from build123d import *

# Parameters (mm, degrees)
SZKIC1_R                               = 4.5
DODANIE_WYCI_GNI_CIE1_DEPTH            = 8
SZKIC23_R                              = 6.5
WYTNIJ_WYCI_GNI_CIE11_DEPTH            = 5.5
SZKIC4_W                               = 8
SZKIC4_H                               = 40
DODANIE_WYCI_GNI_CIE2_DEPTH            = 62.15
DODANIE_WYCI_GNI_CIE3_DEPTH            = 8
WYTNIJ_WYCI_GNI_CIE3_REACH             = 91.171
SZKIC6_R                               = 1.6
SZKIC7_R                               = 3.75
WYTNIJ_WYCI_GNI_CIE4_DEPTH             = 3.5
WYTNIJ_WYCI_GNI_CIE5_REACH             = 97.976
WYTNIJ_WYCI_GNI_CIE5_DIRECTION_2_REACH = 97.976
SZKIC10_R                              = 3
WYTNIJ_WYCI_GNI_CIE6_DEPTH             = 2
WYTNIJ_WYCI_GNI_CIE7_REACH             = 93.888
SZKIC14_W                              = 8
SZKIC14_H                              = 62.15
DODANIE_WYCI_GNI_CIE5_DEPTH            = 78.15
WYTNIJ_WYCI_GNI_CIE9_DEPTH             = 215.763643338
WYTNIJ_WYCI_GNI_CIE9_DEPTH_BACK        = 215.763643338
SZKIC20_W                              = 10
SZKIC20_H                              = 20
WYTNIJ_WYCI_GNI_CIE10_DEPTH            = 5
ZAOKR_GLENIE1_R                        = 10
WYTNIJ_WYCI_GNI_CIE12_REACH            = 213.222
WYTNIJ_WYCI_GNI_CIE12_END_RADIUS       = 5
SZKIC24_R                              = 1.75
WYTNIJ_WYCI_GNI_CIE13_REACH            = 222.301
SZKIC25_R                              = 1.6


with BuildPart() as part:
    # Szkic1 → Dodanie-wyciągnięcie1 (new body)
    with BuildSketch(Plane(origin=(0, 0, 0), x_dir=(1, 0, 0), z_dir=(0, 1, 0))):
        Polygon((-14, -10), (30, -20), (38, -20), (38, 20), (30, 20), (-14, 10), align=None)
        with Locations(Location((0, 0, 0), (0, 0, 270))):
            Circle(SZKIC1_R, mode=Mode.SUBTRACT)
    extrude(amount=DODANIE_WYCI_GNI_CIE1_DEPTH)

    # Szkic23 → Wytnij-wyciągnięcie11 (cut)
    with BuildSketch(Plane.XZ):
        with Locations(Location((0, 0, 0), (0, 0, 270))):
            Circle(SZKIC23_R)
    extrude(amount=-WYTNIJ_WYCI_GNI_CIE11_DEPTH, mode=Mode.SUBTRACT)

    # Szkic4 → Dodanie-wyciągnięcie2 (add)
    with BuildSketch(Plane(origin=(0, 8, 0), x_dir=(1, 0, 0), z_dir=(0, 1, 0))):
        with Locations((34, 0)):
            Rectangle(SZKIC4_W, SZKIC4_H)
    extrude(amount=DODANIE_WYCI_GNI_CIE2_DEPTH)

    # Szkic5 → Dodanie-wyciągnięcie3 (add)
    with BuildSketch(Plane(origin=(0, 70.15, 0), x_dir=(1, 0, 0), z_dir=(0, 1, 0))):
        Polygon((38, -20), (38, 20), (30, 20), (-14, 10), (-14, -10), (30, -20), align=None)
    extrude(amount=DODANIE_WYCI_GNI_CIE3_DEPTH)

    # Szkic6 → Wytnij-wyciągnięcie3 (cut, up to next)
    with BuildSketch(Plane(origin=(0, 78.15, 0), x_dir=(1, 0, 0), z_dir=(0, 1, 0)), mode=Mode.PRIVATE) as wytnij_wyci_gni_cie3_sk1:
        with Locations(Location((-7, 0, 0), (0, 0, 270))):
            Circle(SZKIC6_R)
    wytnij_wyci_gni_cie3_tool1 = extrude(wytnij_wyci_gni_cie3_sk1.sketch, amount=-WYTNIJ_WYCI_GNI_CIE3_REACH, mode=Mode.PRIVATE) & part.part
    # Szkic6 → Wytnij-wyciągnięcie3 (cut, up to next)
    with BuildSketch(Plane(origin=(0, 78.15, 0), x_dir=(1, 0, 0), z_dir=(0, 1, 0)), mode=Mode.PRIVATE) as wytnij_wyci_gni_cie3_sk2:
        with Locations(Location((7, 0, 0), (0, 0, 270))):
            Circle(SZKIC6_R)
    wytnij_wyci_gni_cie3_tool2 = extrude(wytnij_wyci_gni_cie3_sk2.sketch, amount=-WYTNIJ_WYCI_GNI_CIE3_REACH, mode=Mode.PRIVATE) & part.part
    add(wytnij_wyci_gni_cie3_tool1.solids().sort_by_distance((-7, 78.15, 0))[0], mode=Mode.SUBTRACT)
    add(wytnij_wyci_gni_cie3_tool2.solids().sort_by_distance((7, 78.15, 0))[0], mode=Mode.SUBTRACT)

    # Szkic7 → Wytnij-wyciągnięcie4 (cut)
    with BuildSketch(Plane(origin=(0, 78.15, 0), x_dir=(1, 0, 0), z_dir=(0, 1, 0))):
        with Locations(Location((7, 0, 0), (0, 0, 270))):
            Circle(SZKIC7_R)
        with Locations(Location((-7, 0, 0), (0, 0, 270))):
            Circle(SZKIC7_R)
    extrude(amount=-WYTNIJ_WYCI_GNI_CIE4_DEPTH, mode=Mode.SUBTRACT)

    # Wytnij-wyciągnięcie5: up to this plane
    wytnij_wyci_gni_cie5_end = Plane(origin=(30, 78.15, -20), z_dir=(0.22162110358896817, 0, 0.9751328557914598))
    # Szkic9 → Wytnij-wyciągnięcie5 (cut, up to the surface)
    with BuildSketch(Plane(origin=(-14, 0, 0), x_dir=(1, 0, 0), z_dir=(0, 0, 1)), mode=Mode.PRIVATE) as wytnij_wyci_gni_cie5_sk1:
        with BuildLine():
            Line((10.5, 70.15), (17.5, 70.15))
            Line((17.5, 70.15), (17.5, 71.15))
            ThreePointArc((17.5, 71.15), (14, 72.579285786), (10.5, 71.15))
            Line((10.5, 71.15), (10.5, 70.15))
        make_face()
    wytnij_wyci_gni_cie5_tool1 = split(extrude(wytnij_wyci_gni_cie5_sk1.sketch, amount=-WYTNIJ_WYCI_GNI_CIE5_REACH, mode=Mode.PRIVATE), bisect_by=wytnij_wyci_gni_cie5_end, keep=Keep.BOTH, mode=Mode.PRIVATE)
    add(wytnij_wyci_gni_cie5_tool1.solids().sort_by_distance((0, 71.185303, 0))[0], mode=Mode.SUBTRACT)

    # Wytnij-wyciągnięcie5 direction 2: up to this plane
    wytnij_wyci_gni_cie5_direction_2_end = Plane(origin=(-14, 78.15, 10), z_dir=(0.22162110358896792, 0, -0.9751328557914598))
    # Szkic9 → Wytnij-wyciągnięcie5 direction 2 (cut, up to the surface)
    with BuildSketch(Plane(origin=(-14, 0, 0), x_dir=(1, 0, 0), z_dir=(0, 0, 1)), mode=Mode.PRIVATE) as wytnij_wyci_gni_cie5_direction_2_sk1:
        with BuildLine():
            Line((10.5, 70.15), (17.5, 70.15))
            Line((17.5, 70.15), (17.5, 71.15))
            ThreePointArc((17.5, 71.15), (14, 72.579285786), (10.5, 71.15))
            Line((10.5, 71.15), (10.5, 70.15))
        make_face()
    wytnij_wyci_gni_cie5_direction_2_tool1 = split(extrude(wytnij_wyci_gni_cie5_direction_2_sk1.sketch, amount=WYTNIJ_WYCI_GNI_CIE5_DIRECTION_2_REACH, mode=Mode.PRIVATE), bisect_by=wytnij_wyci_gni_cie5_direction_2_end, keep=Keep.BOTH, mode=Mode.PRIVATE)
    add(wytnij_wyci_gni_cie5_direction_2_tool1.solids().sort_by_distance((0, 71.185303, 0))[0], mode=Mode.SUBTRACT)

    # Szkic10 → Wytnij-wyciągnięcie6 (cut)
    with BuildSketch(Plane(origin=(0, 78.15, 0), x_dir=(1, 0, 0), z_dir=(0, 1, 0))):
        with Locations(Location((0, 0, 0), (0, 0, 270))):
            Circle(SZKIC10_R)
    extrude(amount=-WYTNIJ_WYCI_GNI_CIE6_DEPTH, mode=Mode.SUBTRACT)

    # Szkic14 → Wytnij-wyciągnięcie7 (cut, up to next)
    with BuildSketch(Plane.ZY.offset(-30), mode=Mode.PRIVATE) as wytnij_wyci_gni_cie7_sk1:
        with Locations((-16, 39.075)):
            Rectangle(SZKIC14_W, SZKIC14_H)
    wytnij_wyci_gni_cie7_tool1 = extrude(wytnij_wyci_gni_cie7_sk1.sketch, amount=-WYTNIJ_WYCI_GNI_CIE7_REACH, mode=Mode.PRIVATE) & part.part
    # Szkic14 → Wytnij-wyciągnięcie7 (cut, up to next)
    with BuildSketch(Plane.ZY.offset(-30), mode=Mode.PRIVATE) as wytnij_wyci_gni_cie7_sk2:
        with Locations((16, 39.075)):
            Rectangle(SZKIC14_W, SZKIC14_H)
    wytnij_wyci_gni_cie7_tool2 = extrude(wytnij_wyci_gni_cie7_sk2.sketch, amount=-WYTNIJ_WYCI_GNI_CIE7_REACH, mode=Mode.PRIVATE) & part.part
    add(wytnij_wyci_gni_cie7_tool1.solids().sort_by_distance((30, 39.075, -16))[0], mode=Mode.SUBTRACT)
    add(wytnij_wyci_gni_cie7_tool2.solids().sort_by_distance((30, 39.075, 16))[0], mode=Mode.SUBTRACT)

    # Szkic17 → Dodanie-wyciągnięcie5 (add, through all)
    with BuildSketch(Plane.XZ):
        Polygon((38, 20), (196, 12.5), (196, -12.5), (38, -20), (38, -11.990992093), (186, -4.965675637), (186, 4.965675637), (38, 11.990992093), align=None)
    extrude(amount=-DODANIE_WYCI_GNI_CIE5_DEPTH)

    # Szkic18 → Wytnij-wyciągnięcie9 (cut, two sides: drawn at the far end of the back side and taken through both)
    with BuildSketch(Plane(origin=(0, 0, -20), x_dir=(-1, 0, 0), z_dir=(0, 0, -1)).offset(-WYTNIJ_WYCI_GNI_CIE9_DEPTH_BACK)):
        Polygon((-196, 0), (-196, 19.075), (-38, 0), align=None)
        Polygon((-196, 59.075), (-196, 78.15), (-38, 78.15), align=None)
        Polygon((-38, 8), (-186, 25.867721519), (-186, 52.282278481), (-38, 70.15), align=None)
    extrude(amount=WYTNIJ_WYCI_GNI_CIE9_DEPTH + WYTNIJ_WYCI_GNI_CIE9_DEPTH_BACK, mode=Mode.SUBTRACT)

    # Szkic20 → Wytnij-wyciągnięcie10 (cut)
    with BuildSketch(Plane(origin=(196, 0, 0), x_dir=(0, 0, -1), z_dir=(1, 0, 0))):
        with Locations((0, 39.075)):
            Rectangle(SZKIC20_W, SZKIC20_H)
    extrude(amount=-WYTNIJ_WYCI_GNI_CIE10_DEPTH, mode=Mode.SUBTRACT)

    # Zaokrąglenie1
    zaokr_glenie1_edges = [part.edges().sort_by_distance(p)[0] for p in [
        (-14, 4, 10),
        (-14, 4, -10),
        (-14, 74.15, -10),
        (-14, 74.15, 10),
    ]]
    fillet(zaokr_glenie1_edges, radius=ZAOKR_GLENIE1_R)

    # Wytnij-wyciągnięcie12: up to this cylinder (the profile starts outside it)
    wytnij_wyci_gni_cie12_end = Plane(origin=(0, 67.579285786, 0), z_dir=(0, 0, -1)) * Cylinder(WYTNIJ_WYCI_GNI_CIE12_END_RADIUS, 437.444, mode=Mode.PRIVATE)
    # Szkic24 → Wytnij-wyciągnięcie12 (cut, up to the surface)
    with BuildSketch(Plane(origin=(0, 76.15, 0), x_dir=(1, 0, 0), z_dir=(0, 1, 0)), mode=Mode.PRIVATE) as wytnij_wyci_gni_cie12_sk1:
        with Locations(Location((0, 0, 0), (0, 0, 270))):
            Circle(SZKIC24_R)
    wytnij_wyci_gni_cie12_tool1 = extrude(wytnij_wyci_gni_cie12_sk1.sketch, amount=-WYTNIJ_WYCI_GNI_CIE12_REACH, mode=Mode.PRIVATE) - wytnij_wyci_gni_cie12_end
    add(wytnij_wyci_gni_cie12_tool1.solids().sort_by_distance((0, 76.15, 0))[0], mode=Mode.SUBTRACT)

    # Szkic25 → Wytnij-wyciągnięcie13 (cut, up to next)
    with BuildSketch(Plane(origin=(191, 0, 0), x_dir=(0, 0, -1), z_dir=(1, 0, 0)), mode=Mode.PRIVATE) as wytnij_wyci_gni_cie13_sk1:
        with Locations((0, 39.075)):
            Circle(SZKIC25_R)
    wytnij_wyci_gni_cie13_tool1 = extrude(wytnij_wyci_gni_cie13_sk1.sketch, amount=-WYTNIJ_WYCI_GNI_CIE13_REACH, mode=Mode.PRIVATE) & part.part
    add(wytnij_wyci_gni_cie13_tool1.solids().sort_by_distance((191, 39.075, 0))[0], mode=Mode.SUBTRACT)


solid = part.part
Source: CAD feature listing. Evaluate the final solid. Frame: model axes, mm. A direction names the side the tool comes from. Give positions to 0.01 mm unless a question says otherwise; leave off trailing zeros. Write each loop counter-clockwise with the first axis right and the second up, starting at its lowest first coordinate (ties: lowest second). Pieces come first, ordered by that corner, then holes. Notation, with made-up numbers: M 40.25,33.25 L 51.25,33.25 A24 ccw 51.25,69.25 Z; hole C -37,-24.5 d4. An arc over 180 degrees is marked long. Return JSON: item names as keys, results as strings. Group by question number.
1) Cut plane D-D, the plane x = 36. Output: boundary loops of the cut face in (y, z).
2) Ray query, L1, parallel to X at y = 75.65, z = 0; L2, parallel to X at y = 77.45, z = 0; L3, parallel to X at y = 2.05, z = 0. Return the intervals inside material, ascending.
3) Set-up query: faces 1 (the face through (194, 29.075, 0)), 2 (the face through (1.352, 6.732, 4.292)), 3 (the face through (111.655, 13.832, -8.495)). Return all of +Z, -Z, +X, -X, +Y, -Y with unobstructed straight access to the full face (end or side cutting, diameter ignored); none if empty.
4) First-contact query: pin 1 Ø3 at (x, z) = (-7.5, 2.5) entering from -Y; pin 2 Ø4 at (x, y) = (193.5, 44) entering from -Z; pin 3 Ø3 at (x, z) = (0, 0) entering from -Y; pin 4 Ø1.5 at (y, z) = (35.5, -6.5) entering from -X. Flat tips, straight axial feed; report the tip coordinate or a pass-through.
5) Draft query along Z for faces 4 (the face through (-11.756, 74.206, 8.33)), 5 (the face through (21, 70.15, 0)), 6 (the face through (194, 49.075, 0)). Return one class per face: released by +Z, released by -Z, zero draft, split by the parting line, or undercut.
6) Cut plane C-C, the plane y = 67.5. Output: boundary loops of the cut face in (x, z), then the cut area to 3 significant figures.
7) Cut plane B-B, the plane z = 9. Output: boundary loops of the cut face in (x, y) (3 decimals).
8) Cut plane A-A, the plane y = 47. Output: boundary loops of the cut face in (x, z), then the cut area to 3 significant figures.
Data:
{
 "1": {"outline": "M 0,-20 L 8,-20 L 8,-12 L 70.15,-12 L 70.15,-20 L 78.15,-20 L 78.15,20 L 70.15,20 L 70.15,12 L 8,12 L 8,20 L 0,20 Z"},
 "2": {"L1": "x = -14 to -10.75, -3.25 to -1.75, 1.75 to 3.25, 10.75 to 38", "L2": "x = -14 to -10.75, -3.25 to -3, 3 to 3.25, 10.75 to 38", "L3": "x = -14 to -6.5, 6.5 to 38"},
 "3": {"face 1": "+X", "face 2": "-Y", "face 3": "+Y, -Y"},
 "4": {"pin 1": "stops at y = 0", "pin 2": "stops at z = -12.71", "pin 3": "passes through", "pin 4": "stops at x = 30"},
 "5": {"face 4": "released by +Z", "face 5": "zero draft", "face 6": "undercut"},
 "6": {"outline": "M 30,-12 L 38,-12 L 38,12 L 30,12 Z; M 59.95,-18.96 L 126.21,-15.81 L 126.21,-7.8 L 59.95,-10.95 Z; M 59.95,10.95 L 126.21,7.8 L 126.21,15.81 L 59.95,18.96 Z", "area": "1,250 mm²"},
 "7": {"outline": "M -11.159,0 L 38,0 L 38,78.15 L -11.159,78.15 L -11.159,70.15 L -3.5,70.15 L -3.5,71.15 A5 cw 3.5,71.15 L 3.5,70.15 L 30,70.15 L 30,8 L -11.159,8 Z; M 101.01,7.607 L 196,19.075 L 196,59.075 L 101.01,70.543 L 101.01,62.543 L 186,52.282 L 186,25.868 L 101.01,15.607 Z"},
 "8": {"outline": "M 30,-12 L 38,-12 L 38,12 L 30,12 Z; M 186,-12.97 L 196,-12.5 L 196,-5 L 191,-5 L 191,5 L 196,5 L 196,12.5 L 186,12.97 Z", "area": "397 mm²"}
}
